Read the model definition and answer for the solid it produces. Units are mm, in the model's axes. Face numbers are marked on the shaded views. A direction names the side the tool comes from. Round coordinates to 2 decimals unless told otherwise and drop trailing zeros. Write each loop counter-clockwise with the first axis right and the second up, starting at its lowest first coordinate (ties: lowest second). Pieces come first, ordered by that corner, then holes. Notation, with made-up numbers: (35, 0.5) -> (48, 0.5) arc R14 ccw to (48, 10.5) -> close; hole circle Ø9 at (-8, -16). An arc over 180 degrees is marked (long way). Return JSON: item names as keys, results as strings.
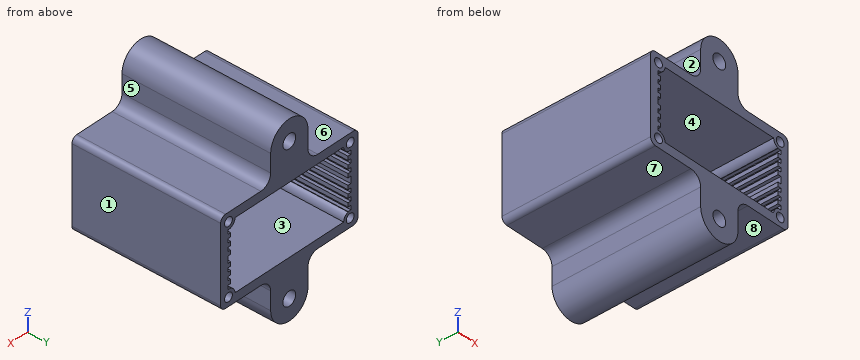
from build123d import *

# Parameters (mm, degrees)
BOSS_EXTRUDE1_DEPTH                        = 69.85
FILLET1_R                                  = 2.54
SKETCH4_R                                  = 3.302
BOSS_EXTRUDE3_DEPTH                        = 69.85
FILLET2_R                                  = 5.08
SKETCH5_R                                  = 3.38963
BOSS_EXTRUDE4_DEPTH                        = 69.85
FILLET1_OF_MIRROR1_R                       = 2.54
FILLET2_OF_MIRROR1_R                       = 5.08
MIRROR2_AT_THE_SECOND_PLANE_COPY_1_SKETC_R = 3.38963
MIRROR2_AT_THE_SECOND_PLANE_COPY_1_DEPTH   = 69.85
SKETCH6_R                                  = 2.032
CUT_EXTRUDE1_DEPTH                         = 90.672163022
MIRROR3_AT_THE_SECOND_PLANE_COPY_1_SKETC_R = 2.032
MIRROR3_AT_THE_SECOND_PLANE_COPY_1_DEPTH   = 90.672163022


with BuildPart() as part:
    # Sketch1 → Boss-Extrude1 (new body)
    with BuildSketch(Plane(origin=(0, 0, 0), x_dir=(1, 0, 0), z_dir=(0, 1, 0))):
        Polygon((30.3657, 16.18107), (-30.3657, 16.18107), (-30.3657, 12.86637), (-31.8135, 12.86637), (-31.8135, 10.98677), (-30.3657, 10.98677), (-30.3657, 9.10717), (-31.8135, 9.10717), (-31.8135, 7.22757), (-30.3657, 7.22757), (-30.3657, 5.34797), (-31.8135, 5.34797), (-31.8135, 3.46837), (-30.3657, 3.46837), (-30.3657, 1.58877), (-31.8135, 1.58877), (-31.8135, 0), (-35.56, 0), (-35.56, 20.32), (35.56, 20.32), (35.56, 0), (31.8135, 0), (31.8135, 1.58877), (30.3657, 1.58877), (30.3657, 3.46837), (31.8135, 3.46837), (31.8135, 5.34797), (30.3657, 5.34797), (30.3657, 7.22757), (31.8135, 7.22757), (31.8135, 9.10717), (30.3657, 9.10717), (30.3657, 10.98677), (31.8135, 10.98677), (31.8135, 12.86637), (30.3657, 12.86637), align=None)
    boss_extrude1 = extrude(amount=BOSS_EXTRUDE1_DEPTH)

    # Fillet1
    fillet1_edges = [part.edges().sort_by_distance(p)[0] for p in [
        (-35.56, 34.925, -20.32),
        (35.56, 34.925, -20.32),
    ]]
    fillet(fillet1_edges, radius=FILLET1_R)

    # Sketch4 → Boss-Extrude3 (add, through all)
    with BuildSketch(Plane(origin=(0, 0, 0), x_dir=(1, 0, 0), z_dir=(0, 1, 0))):
        with BuildLine():
            Line((-9.652, 33.909), (-9.652, 20.32))
            Line((-9.652, 20.32), (9.652, 20.32))
            Line((9.652, 20.32), (9.652, 33.909))
            ThreePointArc((9.652, 33.909), (0, 43.561), (-9.652, 33.909))
        make_face()
        with Locations(Location((0, 33.909, 0), (0, 0, 270))):
            Circle(SKETCH4_R, mode=Mode.SUBTRACT)
    boss_extrude3 = extrude(amount=BOSS_EXTRUDE3_DEPTH)

    # Fillet2
    fillet2_edges = [part.edges().sort_by_distance(p)[0] for p in [
        (-9.652, 34.925, -20.32),
        (9.652, 34.925, -20.32),
    ]]
    fillet(fillet2_edges, radius=FILLET2_R)

    # Sketch5 → Boss-Extrude4 (add)
    with BuildSketch(Plane(origin=(0, 69.85, 0), x_dir=(1, 0, 0), z_dir=(0, 1, 0))):
        with Locations((-31.496, 16.256)):
            Circle(SKETCH5_R)
    boss_extrude4 = extrude(amount=-BOSS_EXTRUDE4_DEPTH)

    # Mirror1: Boss-Extrude1, Boss-Extrude3 across plane
    add(boss_extrude1.mirror(Plane.XY))
    add(boss_extrude3.mirror(Plane.XY))

    # Fillet1 of Mirror1
    fillet1_of_mirror1_edges = [part.edges().sort_by_distance(p)[0] for p in [
        (-35.56, 34.925, 20.32),
        (35.56, 34.925, 20.32),
    ]]
    fillet(fillet1_of_mirror1_edges, radius=FILLET1_OF_MIRROR1_R)

    # Fillet2 of Mirror1
    fillet2_of_mirror1_edges = [part.edges().sort_by_distance(p)[0] for p in [
        (-9.652, 34.925, 20.32),
        (9.652, 34.925, 20.32),
    ]]
    fillet(fillet2_of_mirror1_edges, radius=FILLET2_OF_MIRROR1_R)

    # Mirror2: Boss-Extrude4 across plane
    add(boss_extrude4.mirror(Plane.XY))

    # Mirror2 at the second plane: Boss-Extrude4 across plane
    add(boss_extrude4.mirror(Plane(origin=(0, 0, 0), x_dir=(0, 0, 1), z_dir=(1, 0, 0))))

    # Mirror2 at the second plane copy 1 sketc → Mirror2 at the second plane copy 1 (add)
    with BuildSketch(Plane(origin=(0, 69.85, 0), x_dir=(-1, 0, 0), z_dir=(0, 1, 0))):
        with Locations((-31.496, 16.256)):
            Circle(MIRROR2_AT_THE_SECOND_PLANE_COPY_1_SKETC_R)
    extrude(amount=-MIRROR2_AT_THE_SECOND_PLANE_COPY_1_DEPTH)

    # Sketch6 → Cut-Extrude1 (cut, through all)
    with BuildSketch(Plane(origin=(0, 69.85, 0), x_dir=(1, 0, 0), z_dir=(0, 1, 0))):
        with Locations(Location((-31.496, 16.256, 0), (0, 0, 270))):
            Circle(SKETCH6_R)
    cut_extrude1 = extrude(amount=-CUT_EXTRUDE1_DEPTH, mode=Mode.SUBTRACT)

    # Mirror3: Cut-Extrude1 across plane
    add(cut_extrude1.mirror(Plane.XY), mode=Mode.SUBTRACT)

    # Mirror3 at the second plane: Cut-Extrude1 across plane
    add(cut_extrude1.mirror(Plane(origin=(0, 0, 0), x_dir=(0, 0, 1), z_dir=(1, 0, 0))), mode=Mode.SUBTRACT)

    # Mirror3 at the second plane copy 1 sketc → Mirror3 at the second plane copy 1 (cut, through all)
    with BuildSketch(Plane(origin=(0, 69.85, 0), x_dir=(-1, 0, 0), z_dir=(0, 1, 0))):
        with Locations(Location((-31.496, 16.256, 0), (0, 0, 270))):
            Circle(MIRROR3_AT_THE_SECOND_PLANE_COPY_1_SKETC_R)
    extrude(amount=-MIRROR3_AT_THE_SECOND_PLANE_COPY_1_DEPTH, mode=Mode.SUBTRACT)


solid = part.part
Item 1: Section A-A (x = -19.5) is taken. Give the vertices of the cut face in (y, z), then the cut area to 3 significant figures.
Worked answers:
{"outline": "(0, -20.32) -> (69.85, -20.32) -> (69.85, -16.18) -> (0, -16.18) -> close; (0, 16.18) -> (69.85, 16.18) -> (69.85, 20.32) -> (0, 20.32) -> close", "area": "578 mm2"}
Item 2: Section D-D (y = 60.5) is taken. State how many separate pieces and enclosed holes the cut face has, then the cut area to 3 significant figures.
Worked answers:
{"separate pieces": "1", "enclosed holes": "7", "area": "1,620 mm2"}
Item 3: Section B-B (x = 0) is taken. Give the vertices of the cut face in (y, z), then the cut area to 3 significant figures.
Worked answers:
{"outline": "(0, -43.56) -> (69.85, -43.56) -> (69.85, -37.21) -> (0, -37.21) -> close; (0, -30.61) -> (69.85, -30.61) -> (69.85, -16.18) -> (0, -16.18) -> close; (0, 16.18) -> (69.85, 16.18) -> (69.85, 30.61) -> (0, 30.61) -> close; (0, 37.21) -> (69.85, 37.21) -> (69.85, 43.56) -> (0, 43.56) -> close", "area": "2,900 mm2"}
Item 4: For a pull along X with two mould halves and no side action, classify the marked faces 1, 2, 3 and 4 as released by +X, released by -X, zero draft, split by the parting line, or undercut.
Worked answers:
{"face 1": "released by +X", "face 2": "released by -X", "face 3": "undercut", "face 4": "undercut"}
Item 5: Section C-C (z = -35) is taken. Give the vertices of the cut face in (x, y).
Worked answers:
{"outline": "(-9.59, 0) -> (-3.12, 0) -> (-3.12, 69.85) -> (-9.59, 69.85) -> close; (3.12, 0) -> (9.59, 0) -> (9.59, 69.85) -> (3.12, 69.85) -> close"}
Item 6: A tool of negligible diameter and unlimited length cuts with its end or side. For the marked faces 5, 6, 7 and 8, from which of +Z, -Z, +X, -X, +Y, -Y can it reach the whole face along a straight path? Write none if from no direction.
Worked answers:
{"face 5": "+Z, +X, +Y, -Y", "face 6": "+Z, -X, +Y, -Y", "face 7": "-Z, -X, +Y, -Y", "face 8": "-Z, +X, +Y, -Y"}
Item 7: Straight lines are drawn through the part: L1, parallel to X at y = 19, z = -16; L2, parallel to Z at x = -19, y = 14.5; L3, parallel to X at y = 19, z = -34. For each, find the intervals that lie inside material, in ascending order. Write a range as [from, to].
Worked answers:
{"L1": "x = [-35.56, -33.51], [-29.48, -28.12], [28.12, 29.48], [33.51, 35.56]", "L2": "z = [-20.32, -16.18], [16.18, 20.32]", "L3": "x = [-9.65, -3.3], [3.3, 9.65]"}
Item 8: Flat-ended cylindrical pins translate along their axes: pin 1 (2 mm diameter, centred on x = -2, y = 42.5, fed in from -Z); pin 2 (4.5 mm diameter, centred on y = 46.5, z = 30.5, fed in from -X); pin 3 (1.6 mm diameter, centred on x = -31, y = 20, fed in from -Z). Find the tip coordinate at first contact, or state that the pin passes through.
Worked answers:
{"pin 1": "stops at z = -43.51", "pin 2": "stops at x = -9.65", "pin 3": "stops at z = -20.32"}
